```python
from build123d import *


with BuildPart() as part:
    # Sketch1 → Revolve1 (revolve)
    with BuildSketch(Plane.XY, mode=Mode.PRIVATE) as revolve1_sk:
        with BuildLine():
            Line((30, 186), (43, 186))
            Line((43, 186), (43, 146))
            ThreePointArc((43, 146), (42.529020072, 145.151277561), (42.230898499, 144.22754849))
            Line((42.230898499, 144.22754849), (54.216310346, 21.805127486))
            ThreePointArc((54.216310346, 21.805127486), (54.863243552, 20.518489786), (56.206793881, 20))
            Line((56.206793881, 20), (70, 20))
            Line((70, 20), (70, 0))
            Line((70, 0), (50, 0))
            Line((50, 0), (49.883019474, 1.194872514))
            ThreePointArc((49.883019474, 1.194872514), (49.236086268, 2.481510214), (47.892535939, 3))
            Line((47.892535939, 3), (44, 3))
            Line((44, 3), (30, 146))
            Line((30, 146), (30, 186))
        make_face()
    revolve(revolve1_sk.sketch.rotate(Axis((0, 0, 0), (0, 1, 0)), 90), axis=Axis((0, 0, 0), (0, 1, 0)))


solid = part.part
```
For this review, take the finished solid that the model builds, in its own axes (mm). A direction names the side the tool comes from. Coordinates: 2 decimals unless noted, no trailing zeros. Order: outer loops, then holes, each group sorted by start corner. A loop starts at its lowest first (then second) coordinate and runs counter-clockwise, first axis right, second up. Notation, with made-up numbers: (87.5, 77.25) - (128.5, 77.25) arc R32 cw to (128.5, 113.25) - close; hole circle Ø3 at (89.5, 22.5). An arc over 180 degrees is marked (long way). Answer as a JSON object with one key per item and string values. Group by question number.
1. For faces 1 (the cylindrical face through (68.335, 9.86, 15.175)), 2 (the flat face through (-57, 20, 0)), list the 3-axis set-ups (+Z, -Z, +X, -X, +Y, -Y) from which the entire face can be reached by the end or side of a thin tool; tool diameter is ignored.
2. We need section A-A on z = 0. State the section outline as (x, y) points.
3. Clearance check with flat-ended pins moving along their axes: P1, Ø6, axis at y = 73.5, z = -15, coming from the +X side; P2, Ø10, axis at y = 66, z = -23.5, coming from the -X side; P3, Ø8, axis at y = 87, z = 15.5, coming from the +X side. State where each tip first meets the part, or that it passes through.
4. We need section C-C on y = 52.5. State the section outline as (x, z) points.
5. We need section D-D on y = 159. State the section outline as (x, z) points, then the cut area to 3 significant figures.
6. For probe 1 along X at (y, z) = (174, 0); probe 2 along X at (y, z) = (125, 24.5); probe 3 along Z at (x, y) = (-11.5, 153), list the stretches that pass through material, from the lowest coordinate up.
7. The part is to be moulded in two halves that separate along Z. For faces 3 (the flat face through (39, 3, -21)), 4 (the cylindrical face through (-42.634, 165.72, 5.598)), 5 (the cylindrical face through (-25.296, 166.28, -16.128)), 6 (the flat face through (-17, 0, 48)), say which applies: pulls with the +Z half, pulls with the -Z half, needs draft (parallel to the pull), parting line crosses it, or undercut.
8. We need section B-B on x = 0. State the section outline as (y, z) points, then the cut area to 3 significant figures.
Final values:
{
 "1": {"face 1": "+Y, -Y", "face 2": "+Y"},
 "2": {"outline": "(-70, 0) - (-50, 0) - (-49.88, 1.19) arc R2 cw to (-47.89, 3) - (-44, 3) - (-30, 146) - (-30, 186) - (-43, 186) - (-43, 146) arc R5 cw to (-42.23, 144.23) - (-54.22, 21.81) arc R2 cw to (-56.21, 20) - (-70, 20) - close; (30, 146) - (44, 3) - (47.89, 3) arc R2 cw to (49.88, 1.19) - (50, 0) - (70, 0) - (70, 20) - (56.21, 20) arc R2 cw to (54.22, 21.81) - (42.23, 144.23) arc R5 cw to (43, 146) - (43, 186) - (30, 186) - close"},
 "3": {"P1": "x = 47.73", "P2": "x = -46.4", "P3": "x = 46.51"},
 "4": {"outline": "circle Ø102.42 at (0, 0); hole circle Ø78.31 at (0, 0)"},
 "5": {"outline": "circle Ø86 at (0, 0); hole circle Ø60 at (0, 0)", "area": "2,980 mm²"},
 "6": {"probe 1": "-43 to -30, 30 to 43", "probe 2": "-36.68 to -20.67, 20.67 to 36.68", "probe 3": "-41.43 to -27.71, 27.71 to 41.43"},
 "7": {"face 3": "undercut", "face 4": "parting line crosses it", "face 5": "undercut", "face 6": "needs draft"},
 "8": {"outline": "(0, -70) - (20, -70) - (20, -56.21) arc R2 cw to (21.81, -54.22) - (144.23, -42.23) arc R5 cw to (146, -43) - (186, -43) - (186, -30) - (146, -30) - (3, -44) - (3, -47.89) arc R2 cw to (1.19, -49.88) - (0, -50) - close; (0, 50) - (1.19, 49.88) arc R2 cw to (3, 47.89) - (3, 44) - (146, 30) - (186, 30) - (186, 43) - (146, 43) arc R5 cw to (144.23, 42.23) - (21.81, 54.22) arc R2 cw to (20, 56.21) - (20, 70) - (0, 70) - close", "area": "5,120 mm²"}
}
